Geometry check sheet. Reference: drawing and pictorial views, mm from the part's lowest x, y, z. A direction names the side the tool comes from. Give positions to 0.01 mm unless a question says otherwise; leave off trailing zeros. Write each loop counter-clockwise with the first axis right and the second up, starting at its lowest first coordinate (ties: lowest second). Pieces come first, ordered by that corner, then holes. Notation, with made-up numbers: (68.5, -5) -> (101.5, -5) arc R20 ccw to (101.5, 11) -> close; hole circle Ø11 at (32.25, 51). An arc over 180 degrees is marked (long way). Answer as CSV lines item,"result".
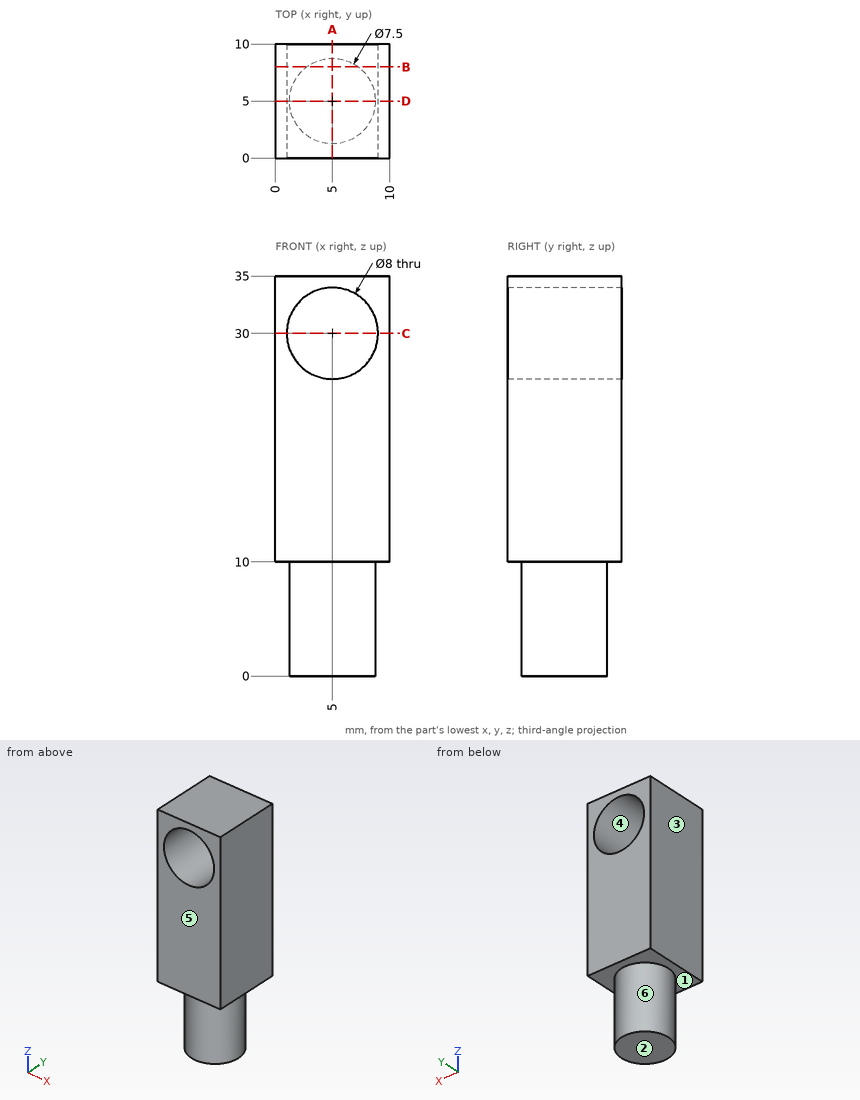
1) Section check A-A (x = 5). Record the boundary of the cut face in (y, z).
Reported:
outline,"(0, 10) -> (1.25, 10) -> (1.25, 0) -> (8.75, 0) -> (8.75, 10) -> (10, 10) -> (10, 26) -> (0, 26) -> close; (0, 34) -> (10, 34) -> (10, 35) -> (0, 35) -> close"
2) Section check C-C (z = 30). Record the boundary of the cut face in (x, y), and give its area (3 significant figures).
Reported:
outline,"(0, 0) -> (1, 0) -> (1, 10) -> (0, 10) -> close; (9, 0) -> (10, 0) -> (10, 10) -> (9, 10) -> close"
area,"20.0 mm²"
3) Draft check along X on the marked faces 3, 4, 5 and 6. Enter one of: +X half, -X half, draft (parallel to the pull), parting line (faces both ways), or undercut.
Reported:
face 3,"-X half"
face 4,"undercut"
face 5,"draft"
face 6,"parting line"
4) Section check D-D (y = 5). Record the boundary of the cut face in (x, z).
Reported:
outline,"(0, 10) -> (1.25, 10) -> (1.25, 0) -> (8.75, 0) -> (8.75, 10) -> (10, 10) -> (10, 35) -> (0, 35) -> close; hole circle Ø8 at (5, 30)"
5) Scan lines: line 1 along Z through (x, y) = (5, 5.75); line 2 along Z through (x, y) = (9.25, 4); line 3 along Z through (x, y) = (2.25, 3.5). Record each from-to range of solid material in increasing order.
Reported:
line 1,"0 to 26, 34 to 35"
line 2,"10 to 35"
line 3,"0 to 27.1, 32.9 to 35"
6) Section check B-B (y = 8). Record the boundary of the cut face in (x, z), and give its area (3 significant figures).
Reported:
outline,"(0, 10) -> (2.75, 10) -> (2.75, 0) -> (7.25, 0) -> (7.25, 10) -> (10, 10) -> (10, 35) -> (0, 35) -> close; hole circle Ø8 at (5, 30)"
area,"245 mm²"
7) Tool access check on the marked faces 1 and 2. Record the directions out of +Z, -Z, +X, -X, +Y, -Y that give a thin tool (end or side, any length) a straight path to the whole face; none if there is none.
Reported:
face 1,"-Z"
face 2,"-Z, +X, -X, +Y, -Y"
